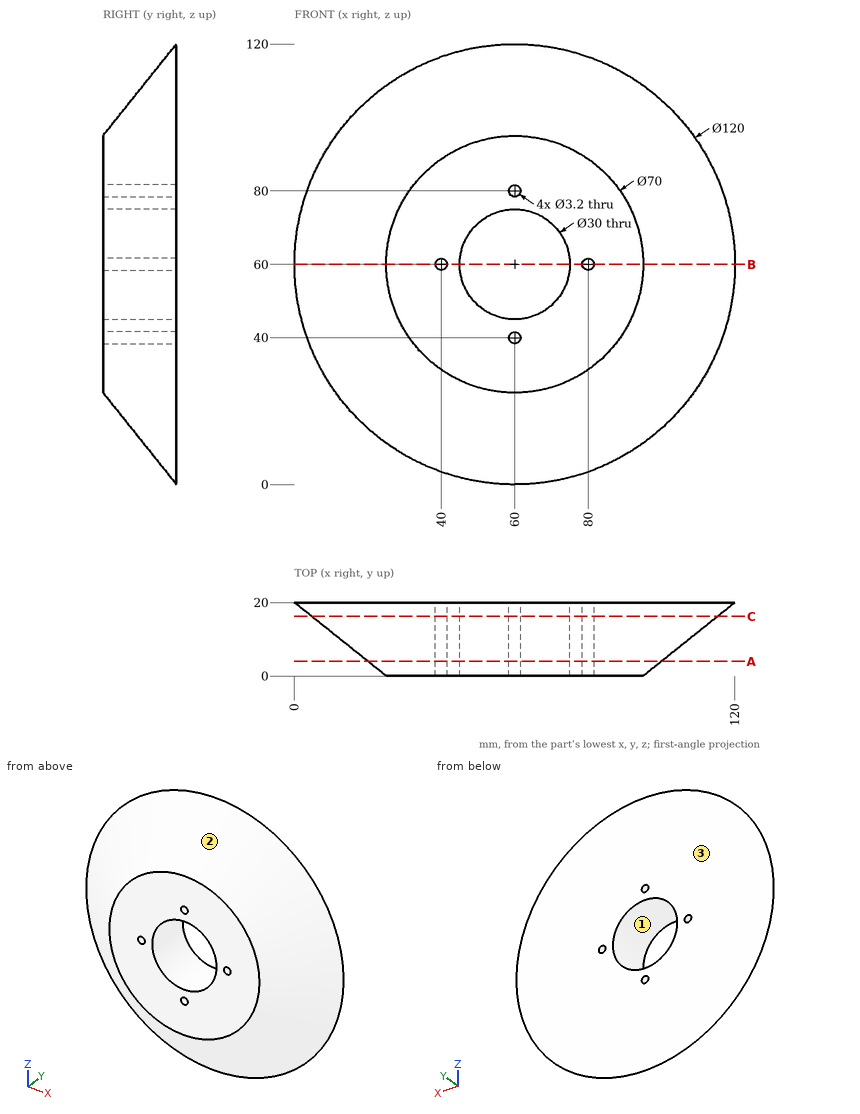
The figure shows three views and two pictorial views of one solid part (mm, origin at its lowest corner). Answer the questions. Give positions to 0.01 mm unless a question says otherwise; leave off trailing zeros. Write each loop counter-clockwise with the first axis right and the second up, starting at its lowest first coordinate (ties: lowest second). Pieces come first, ordered by that corner, then holes. Notation, with made-up numbers: (56, -9) -> (103, -9) arc R17 cw to (103, -2) -> close; hole circle Ø8 at (85.25, 32.25). An arc over 180 degrees is marked (long way). Use one line per item in the form item = value.
1) Section C-C on y = 16.25 is taken. Write down the section's boundary in (x, z) (1 decimal).
Result:
outline = circle Ø110.6 at (60, 60); hole circle Ø3.2 at (40, 60); hole circle Ø30 at (60, 60); hole circle Ø3.2 at (60, 40); hole circle Ø3.2 at (60, 80); hole circle Ø3.2 at (80, 60)
2) Section A-A on y = 4 is taken. Write down the section's boundary in (x, z).
Result:
outline = circle Ø80 at (60, 60); hole circle Ø3.2 at (40, 60); hole circle Ø30 at (60, 60); hole circle Ø3.2 at (60, 40); hole circle Ø3.2 at (60, 80); hole circle Ø3.2 at (80, 60)
3) Section B-B on z = 60 is taken. Count the separate pieces of the cut face and the enclosed holes in it, plus the area to 3 significant figures.
Result:
separate_pieces = 4
enclosed_holes = 0
area = 1,170 mm²
4) For a pull along Z with two mould halves and no side action, classify the marked faces 1, 2 and 3 as +Z half, -Z half, draft (parallel to the pull), parting line (faces both ways), or undercut.
Result:
face_1 = undercut
face_2 = parting line
face_3 = draft
5) Each of these flat-tipped pins is pushed along its axis until it touches: P1, Ø3, axis at x = 64.5, y = 3.5, coming from the +Z side; P2, Ø6, axis at x = 69, y = 16, coming from the -Z side; P3, Ø8, axis at y = 9.5, z = 64.5, coming from the -X side. Where does it stop, or does it pass through?
Result:
P1 = 101.01
P2 = 1.92
P3 = 8.31
6) Straight lines are drawn through the part: probe 1 along X at (y, z) = (15, 80); probe 2 along X at (y, z) = (4.75, 80); probe 3 along Z at (x, y) = (58, 1.25). For each, find the intervals that lie inside material, in ascending order.
Result:
probe_1 = 10.11 to 58.4, 61.6 to 109.89
probe_2 = 24.28 to 58.4, 61.6 to 95.72
probe_3 = 23.49 to 45.13, 74.87 to 96.51
